from build123d import *

# Parameters (mm, degrees)
SKETCH1_R           = 2.6924
BOSS_EXTRUDE1_DEPTH = 11.43


with BuildPart() as part:
    # Sketch1 → Boss-Extrude1 (new body)
    with BuildSketch(Plane(origin=(0, 0, 0), x_dir=(0, 0, -1), z_dir=(1, 0, 0))):
        with BuildLine():
            Line((-17.248379124, 31.777583848), (-18.961429782, 34.60046561))
            add(Edge.make_bspline(
                [(-18.961429782, 34.60046561), (-23.58056, 31.333147995), (-34.069402621, 23.636456001)],
                knots=[0, 0, 0, 1, 1, 1], degree=2))
            ThreePointArc((-34.069402621, 23.636456001), (-38.936367326, 17.418147401), (-35.185150313, 24.366750009))
            add(Edge.make_bspline(
                [(-19.655711627, 35.744550608), (-24.45282225, 32.833449755), (-33.10684296, 27.542000808), (-35.185150313, 24.366750009)],
                knots=[0, 0, 0, 0, 1, 1, 1, 1], degree=3))
            ThreePointArc((-19.655711627, 35.744550608), (40.669779942, -3.160521672), (-24.941927486, -32.278787942))
            add(Edge.make_bspline(
                [(-24.941927486, -32.278787942), (-28.90001234, -29.501694158), (-35.285813522, -22.100360431), (-37.707971273, -17.877142062)],
                knots=[0, 0, 0, 0, 1, 1, 1, 1], degree=3))
            ThreePointArc((-37.707971273, -17.877142062), (-42.120851326, -11.328768455), (-36.669004411, -17.041217359))
            add(Edge.make_bspline(
                [(-24.172835506, -31.182630753), (-28.247821961, -28.091199741), (-32.832203399, -21.809959197), (-36.669004411, -17.041217359)],
                knots=[0, 0, 0, 0, 1, 1, 1, 1], degree=3))
            Line((-24.172835506, -31.182630753), (-22.276314881, -28.479592921))
            ThreePointArc((-22.276314881, -28.479592921), (36.03168324, -3.006529649), (-17.248379124, 31.777583848))
        make_face()
        with Locations((-36.766350845, 20.733511971)):
            Circle(SKETCH1_R, mode=Mode.SUBTRACT)
        with Locations((-39.636960779, -14.415984273)):
            Circle(SKETCH1_R, mode=Mode.SUBTRACT)
    extrude(amount=BOSS_EXTRUDE1_DEPTH)


solid = part.part
The model under review builds one solid part; all positions refer to its coordinate system, in mm. A direction names the side the tool comes from. Coordinates: 2 decimals unless noted, no trailing zeros. Loops run counter-clockwise (first coordinate to the right, second up) from the corner with the lowest first, then second, coordinate; pieces in that order, holes last. Notation, with made-up numbers: M 75.25,-13 L 126.25,-13 A27 cw 126.25,4 Z; hole C 44,-12.75 d3. An arc over 180 degrees is marked long. Put each result on its own line as item: value. Start each with the question number.
Q1. Add section A-A (z = 0). Write out the cut boundary in (x, y).
Q2. The part is to be moulded in two halves that separate along Z. For faces 3 (the cylindrical face through (5.635, -1.934, -40.747)), 4 (the cylindrical face through (5.635, -11.435, 42.247)), 5 (the flat face through (11.43, -2.8, -36.3)), say which applies: +Z half, -Z half, draft (parallel to the pull), parting line (faces both ways), or undercut.
Q3. Clearance check with flat-ended pins moving along their axes: pin 1 (6 mm diameter, centred on y = -14.42, z = 39.64, fed in from -X); pin 2 (1.5 mm diameter, centred on x = 8, z = -16, fed in from +Y); pin 3 (1 mm diameter, centred on x = 1.5, z = -31, fed in from +Y); pin 4 (1 mm diameter, centred on x = 8.5, z = 3, fed in from -Y). State where each tip first meets the part, or that it passes through.
Q4. Add section C-C (z = -8.5). Write out the cut boundary in (x, y), and give its area (3 significant figures).
Q5. Add section B-B (y = 22). Write out the cut boundary in (x, z), and give its area (3 significant figures).
Q6. For faces 1 (the flat face through (5.63, -29.85, 23.24)), 2 (the flat face through (0, -2.8, -36.3)), list the 3-axis set-ups (+Z, -Z, +X, -X, +Y, -Y) from which the entire face can be reached by the end or side of a thin tool; tool diameter is ignored.
Q7. Wall thickness on line 1 (Y direction, x = 8.5, z = 0); line 2 (Z direction, x = 8, y = -12); line 3 (Y direction, x = 5.5, z = -23.5): over which ranges is each line inside the solid? List them lowest first.
Q8. Add section D-D (y = 0). Write out the cut boundary in (x, z).
Answers:
1. outline: M 0,-40.79 L 11.43,-40.79 L 11.43,-36.16 L 0,-36.16 Z; M 0,36.16 L 11.43,36.16 L 11.43,40.79 L 0,40.79 Z
2. face 3: parting line
2. face 4: undercut
2. face 5: draft
3. pin 1: stops at x = 0
3. pin 2: stops at y = 37.83
3. pin 3: stops at y = 27.09
3. pin 4: stops at y = -40.72
4. outline: M 0,-39.9 L 11.43,-39.9 L 11.43,-35.14 L 0,-35.14 Z; M 0,35.14 L 11.43,35.14 L 11.43,39.9 L 0,39.9 Z
4. area: 109 mm^2
5. outline: M 0,-34.35 L 11.43,-34.35 L 11.43,-28.69 L 0,-28.69 Z; M 0,33.01 L 11.43,33.01 L 11.43,34.39 L 0,34.39 Z; M 0,39.14 L 11.43,39.14 L 11.43,40.52 L 0,40.52 Z
5. area: 96.2 mm^2
6. face 1: +X, -X
6. face 2: +Z, -Z, -X, +Y, -Y
7. line 1: y = -40.79 to -36.16, 36.16 to 40.79
7. line 2: z = -38.99 to -34.11, 36.5 to 38.45, 40.83 to 42.78
7. line 3: y = -33.34 to -27.48, 27.48 to 33.34
8. outline: M 0,-40.79 L 11.43,-40.79 L 11.43,-36.16 L 0,-36.16 Z
